from build123d import *

# Parameters (mm, degrees)
F0_W     = 300
F0_H     = 15
F0_R     = 5
F1_DEPTH = 10
F2_DEPTH = 25
F4_W     = 10
F4_H     = 15
F5_DEPTH = 250


with BuildPart() as f1:
    # F0 (on Front) → F1 (new body)
    with BuildSketch(Plane.XZ):
        Rectangle(F0_W, F0_H)
        with Locations((-125, 0)):
            Circle(F0_R, mode=Mode.SUBTRACT)
        with Locations((125, 0)):
            Circle(F0_R, mode=Mode.SUBTRACT)
    extrude(amount=F1_DEPTH)

    # F0 (on Front) → F2 (join)
    with BuildSketch(Plane.XZ):
        with Locations((-125, 0)):
            Circle(F0_R)
        with Locations((125, 0)):
            Circle(F0_R)
    extrude(amount=F2_DEPTH)

    # F4 (on offset) → F5 (join)
    with BuildSketch(Plane(origin=(-150, 0, 0), x_dir=(0, -1, 0), z_dir=(-1, 0, 0))):
        with Locations((4.988082091, 0)):
            Rectangle(F4_W, F4_H)
    extrude(amount=F5_DEPTH)


solid = f1.part
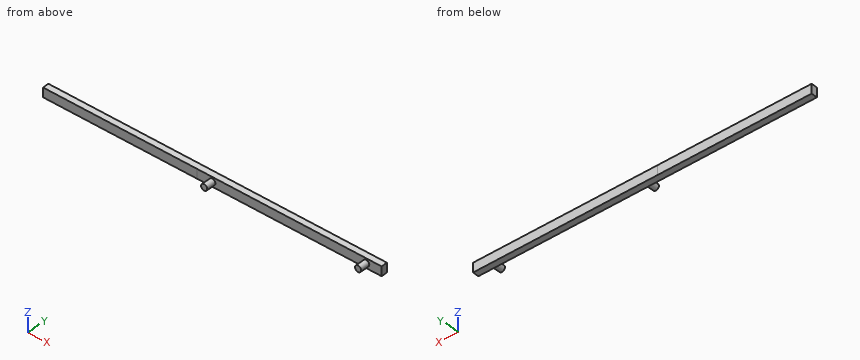
Geometry check sheet. Reference: the model listing, model coordinates, mm. Give positions to 0.01 mm unless a question says otherwise; leave off trailing zeros. Write each loop counter-clockwise with the first axis right and the second up, starting at its lowest first coordinate (ties: lowest second). Pieces come first, ordered by that corner, then holes.
1) Cross-section at C-C (x = 125). Record the boundary of the cut face in (y, z).
Values follow:
outline: (-25, -5) - (-10, -5) - (-10, -7.5) - (0, -7.5) - (0, 7.5) - (-10, 7.5) - (-10, 5) - (-25, 5) - close
2) Cross-section at A-A (y = -16.5). Record the boundary of the cut face in (x, z).
Values follow:
outline: circle Ø10 at (-125, 0); circle Ø10 at (125, 0)
3) Cross-section at D-D (x = -115). Record the boundary of the cut face in (y, z), plus the area to 3 significant figures.
Values follow:
outline: (-10, -7.5) - (0, -7.5) - (0, 7.5) - (-10, 7.5) - close
area: 150 mm2
4) Thickness scan on line 1 (X direction, y = -10.5, z = -0.25); line 2 (Y direction, x = 102, z = 0.25); line 3 (X direction, y = -17.5, z = -3.25). Record the ranges inside material, lowest first.
Values follow:
line 1: x = -129.99 to -120.01, 120.01 to 129.99
line 2: y = -10 to 0
line 3: x = -128.8 to -121.2, 121.2 to 128.8
5) Go/stop test with flat-tipped pins: pin 1 Ø6 at (y, z) = (-22.5, 0.5) entering from +X; pin 2 Ø10 at (x, y) = (-20, -17.5) entering from +Z (3 decimals); pin 3 Ø1 at (y, z) = (-12.5, 2.5) entering from +X; pin 4 Ø5 at (y, z) = (-14.5, -4) entering from -X. Record where each tip stops, or that it passes through.
Values follow:
pin 1: stops at x = 130
pin 2: passes through
pin 3: stops at x = 129.58
pin 4: stops at x = -129.77
